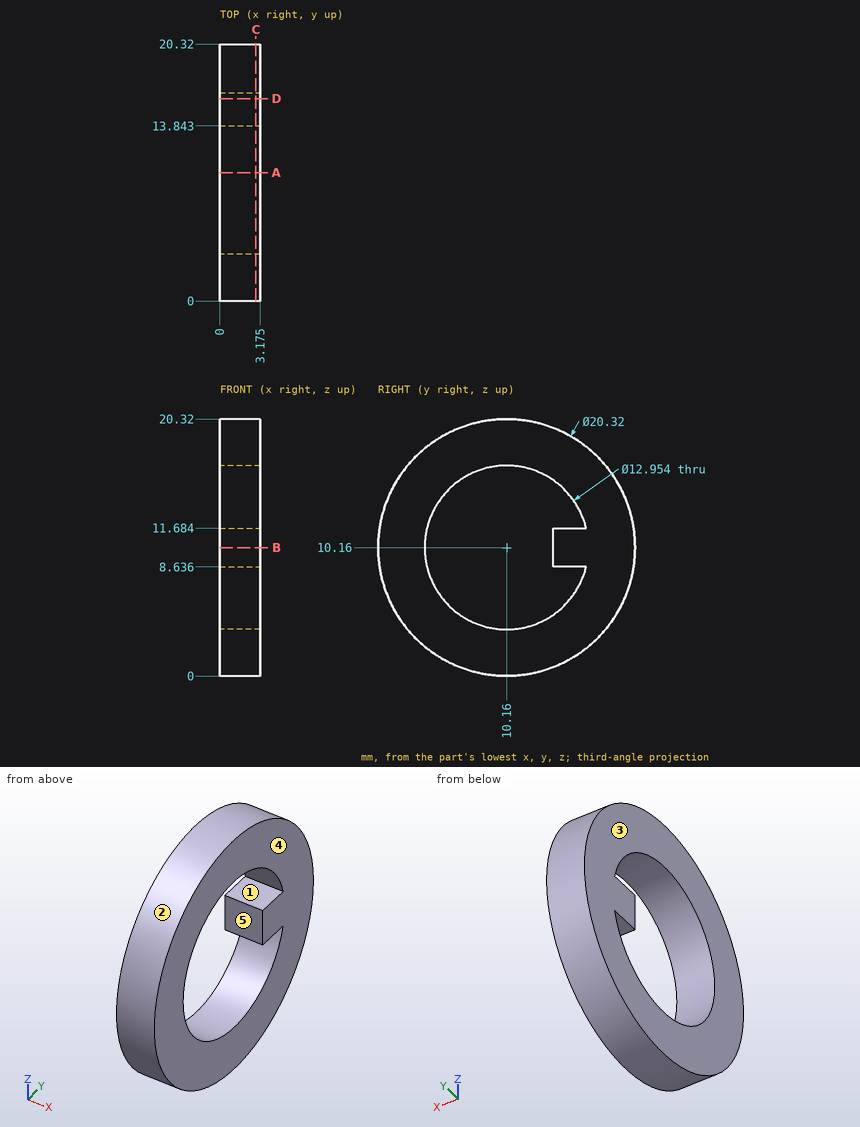
For this review, use the dimensioned drawing (mm, ordinates from the lowest corner) and the shaded views. A direction names the side the tool comes from. Coordinates: 2 decimals unless noted, no trailing zeros. Loops run counter-clockwise (first coordinate to the right, second up) from the corner with the lowest first, then second, coordinate; pieces in that order, holes last. Notation, with made-up numbers: (59, -30) -> (91, -30) arc R7 cw to (91, -22) -> close; hole circle Ø5 at (-16, 25). An arc over 180 degrees is marked (long way). Use a Markdown table: item, result. Add a question column.
1. Draft analysis for pull direction Z (two halves, no side actions). For the marked faces 1, 2 and 3, state which applies: pulls with the +Z half, pulls with the -Z half, needs draft (parallel to the pull), parting line crosses it, or undercut.
2. Clearance check with flat-ended pins moving along their axes: pin 1 Ø8 at (y, z) = (6.5, 17) entering from -X; pin 2 Ø1.5 at (y, z) = (13, 10.5) entering from -X; pin 3 Ø1 at (x, y) = (1, 5) entering from +Z. State where each tip first meets the part, or that it passes through.
3. Add section C-C on x = 2.85. Write out the cut boundary in (y, z).
4. Machinability: for the marked faces 4 and 5, which of the approach directions +Z, -Z, +X, -X, +Y, -Y give a long, thin tool a straight path to every point of the face, cutting with its end or side? Answer none if there is none.
5. Add section D-D on y = 16. Write out the cut boundary in (x, z) (3 decimals), plus the area to 3 significant figures.
6. To check wall thickness, follow line 1 (Z direction, x = 2.1, y = 10.16); line 2 (Y direction, x = 0.95, z = 10.16); line 3 (Z direction, x = 1.35, y = 7.5). State the ranges of each line that lie inside material, in increasing order.
7. Add section A-A on y = 10.16. Write out the cut boundary in (x, z) (3 decimals).
8. Add section B-B on z = 10.16. Write out the cut boundary in (x, y) (3 decimals).
Returned:
| question | item | result |
|---|---|---|
| 1 | face 1 | undercut |
| 1 | face 2 | parting line crosses it |
| 1 | face 3 | needs draft |
| 2 | pin 1 | stops at x = 0 |
| 2 | pin 2 | passes through |
| 2 | pin 3 | stops at z = 19.19 |
| 3 | outline | circle Ø20.32 at (10.16, 10.16); hole (13.84, 8.64) -> (13.84, 11.68) -> (16.46, 11.68) arc R6.48 ccw (long way) to (16.46, 8.64) -> close |
| 4 | face 4 | +Z, -Z, +X, +Y, -Y |
| 4 | face 5 | +X, -X |
| 5 | outline | (0, 1.846) -> (3.175, 1.846) -> (3.175, 7.359) -> (0, 7.359) -> close; (0, 8.636) -> (3.175, 8.636) -> (3.175, 11.684) -> (0, 11.684) -> close; (0, 12.961) -> (3.175, 12.961) -> (3.175, 18.474) -> (0, 18.474) -> close |
| 5 | area | 44.7 mm² |
| 6 | line 1 | z = 0 to 3.68, 16.64 to 20.32 |
| 6 | line 2 | y = 0 to 3.68, 13.84 to 20.32 |
| 6 | line 3 | z = 0.35 to 4.25, 16.07 to 19.97 |
| 7 | outline | (0, 0) -> (3.175, 0) -> (3.175, 3.683) -> (0, 3.683) -> close; (0, 16.637) -> (3.175, 16.637) -> (3.175, 20.32) -> (0, 20.32) -> close |
| 8 | outline | (0, 0) -> (3.175, 0) -> (3.175, 3.683) -> (0, 3.683) -> close; (0, 13.843) -> (3.175, 13.843) -> (3.175, 20.32) -> (0, 20.32) -> close |
